The listing builds one solid part. Answer for the finished solid, in the listing's coordinates (mm). Round coordinates to 2 decimals unless told otherwise and drop trailing zeros. Order: outer loops, then holes, each group sorted by start corner. A loop starts at its lowest first (then second) coordinate and runs counter-clockwise, first axis right, second up. Notation, with made-up numbers: M 43,77 L 87,77 A16 ccw 87,100 Z; hole C 84,73 d5. An arc over 180 degrees is marked long. Write item = value, one per line. Start each with the question number.
(1) Each of these flat-tipped pins is pushed along its axis until it touches: pin 1 (11 mm diameter, centred on x = -1, z = -160.25, fed in from -Y); pin 2 (2 mm diameter, centred on y = 0.5, z = 167.5, fed in from +X); pin 3 (1.5 mm diameter, centred on x = -12.5, y = 1.5, fed in from +Z); pin 4 (1.5 mm diameter, centred on x = 175, y = 2, fed in from -Z). Where does it stop, or does it pass through?
(2) For a pull along Z with two mould halves and no side action, classify faces 1 (the face through (103.257, 2.535, 9.442)), 2 (the face through (-3, 5, 7)) as released by +Z, released by -Z, zero draft, split by the parting line, or undercut.
(3) A cutting plane is placed at A-A, the plane z = -127.75. Determine the outline of the cut face in (x, y), and give its area (3 significant figures).
(4) A cutting plane is placed at D-D, the plane x = 79. Determine the outline of the cut face in (y, z).
(5) A cutting plane is placed at B-B, the plane x = -1. Determine the outline of the cut face in (y, z), and give its area (3 significant figures).
(6) Straight lines are drawn through the part: probe 1 along Z at (x, y) = (-1, 3.7); probe 2 along X at (y, z) = (2.2, 239); probe 3 along Z at (x, y) = (110.25, 1.55). For each, find the intervals that lie inside material, in ascending order. Write a range as from..to.
(7) A cutting plane is placed at C-C, the plane z = 42.25. Determine the outline of the cut face in (x, y).
from build123d import *

# Parameters (mm, degrees)
SKETCH1_W                    = 458
SKETCH1_H                    = 458
BOSS_EXTRUDE1_DEPTH          = 5
SKETCH2_W                    = 85
SKETCH2_H                    = 85
CUT_EXTRUDE1_DEPTH           = 324.893501015
SKETCH4_W                    = 50
SKETCH4_H                    = 20
BOSS_EXTRUDE2_DEPTH          = 5
FILLET1_R                    = 5
FILLET2_R                    = 5
F_5_0_5_DIAMETER_HOLE1_D     = 5
F_5_0_5_DIAMETER_HOLE1_DEPTH = 38
F_5_0_5_DIAMETER_HOLE1_TIP   = 1.502151548
F_14_0_14_DIAMETER_HOLE1_D   = 14


with BuildPart() as part:
    # Sketch1 → Boss-Extrude1 (new body)
    with BuildSketch(Plane(origin=(0, 0, 0), x_dir=(1, 0, 0), z_dir=(0, 1, 0))):
        Rectangle(SKETCH1_W, SKETCH1_H)
    extrude(amount=BOSS_EXTRUDE1_DEPTH)

    # Sketch2 → Cut-Extrude1 (cut, through all)
    with BuildSketch(Plane(origin=(0, 5, 0), x_dir=(1, 0, 0), z_dir=(0, 1, 0))):
        with Locations((-186.5, 186.5)):
            Rectangle(SKETCH2_W, SKETCH2_H)
        with Locations((186.5, 186.5)):
            Rectangle(SKETCH2_W, SKETCH2_H)
        with Locations((186.5, -186.5)):
            Rectangle(SKETCH2_W, SKETCH2_H)
        with Locations((-186.5, -186.5)):
            Rectangle(SKETCH2_W, SKETCH2_H)
    extrude(amount=-CUT_EXTRUDE1_DEPTH, mode=Mode.SUBTRACT)

    # Sketch4 → Boss-Extrude2 (add)
    with BuildSketch(Plane(origin=(0, 5, 0), x_dir=(1, 0, 0), z_dir=(0, 1, 0))):
        with Locations((-119, -239)):
            Rectangle(SKETCH4_W, SKETCH4_H)
        with Locations((119, -239)):
            Rectangle(SKETCH4_W, SKETCH4_H)
    extrude(amount=-BOSS_EXTRUDE2_DEPTH)

    # Fillet1
    fillet1_edges = [part.edges().sort_by_distance(p)[0] for p in [
        (-144, 2.5, 144),
        (144, 2.5, 144),
        (144, 2.5, -144),
        (-144, 2.5, -144),
        (-94, 2.5, 229),
        (94, 2.5, 229),
    ]]
    fillet(fillet1_edges, radius=FILLET1_R)

    # Fillet2
    fillet2_edges = [part.edges().sort_by_distance(p)[0] for p in [
        (-229, 2.5, 144),
        (229, 2.5, 144),
        (229, 2.5, -144),
        (144, 2.5, -229),
        (-229, 2.5, -144),
        (-144, 2.5, -229),
        (-144, 2.5, 249),
        (-94, 2.5, 249),
        (144, 2.5, 249),
        (94, 2.5, 249),
    ]]
    fillet(fillet2_edges, radius=FILLET2_R)

    # Ø5.0 (5) Diameter Hole1
    with Locations(Plane(origin=(0, 5, 0), x_dir=(1, 0, 0), z_dir=(0, 1, 0))):
        with Locations((-119, -239), (119, -239)):
            Hole(F_5_0_5_DIAMETER_HOLE1_D / 2, depth=F_5_0_5_DIAMETER_HOLE1_DEPTH)
            with Locations((0, 0, -(F_5_0_5_DIAMETER_HOLE1_DEPTH + F_5_0_5_DIAMETER_HOLE1_TIP / 2))):  # 118° drill point
                Cone(0, F_5_0_5_DIAMETER_HOLE1_D / 2, F_5_0_5_DIAMETER_HOLE1_TIP, mode=Mode.SUBTRACT)

    # Ø14.0 (14) Diameter Hole1 (through all)
    with Locations(Plane(origin=(0, 0, 0), x_dir=(-1, 0, 0), z_dir=(0, -1, 0))):
        with Locations((112.25, 127.75), (112.25, -9.75), (1, 160.25), (-110.25, 127.75), (-110.25, -9.75), (1, -42.25)):
            Hole(F_14_0_14_DIAMETER_HOLE1_D / 2)


solid = part.part
Reported:
q1.pin_1 = through
q1.pin_2 = 144
q1.pin_3 = 229
q1.pin_4 = -144
q2.face_1 = undercut
q2.face_2 = zero draft
q3.outline = M -229,0 L -119.25,0 L -119.25,5 L -229,5 Z; M -105.25,0 L 103.25,0 L 103.25,5 L -105.25,5 Z; M 117.25,0 L 229,0 L 229,5 L 117.25,5 Z
q3.area = 2,150 mm²
q4.outline = M 0,-229 L 5,-229 L 5,229 L 0,229 Z
q5.outline = M 0,-229 L 5,-229 L 5,-167.25 L 0,-167.25 Z; M 0,-153.25 L 5,-153.25 L 5,35.25 L 0,35.25 Z; M 0,49.25 L 5,49.25 L 5,229 L 0,229 Z
q5.area = 2,150 mm²
q6.probe_1 = -229..-167.25, -153.25..35.25, 49.25..229
q6.probe_2 = -144..-121.5, -116.5..-94, 94..116.5, 121.5..144
q6.probe_3 = -229..-134.75, -120.75..2.75, 16.75..249
q7.outline = M -229,0 L -8,0 L -8,5 L -229,5 Z; M 6,0 L 229,0 L 229,5 L 6,5 Z
